Model file for the job. Use its own axes, mm. Face numbers are marked on the shaded views. A direction names the side the tool comes from. Give positions to 0.01 mm unless a question says otherwise; leave off trailing zeros. Loops run counter-clockwise (first coordinate to the right, second up) from the corner with the lowest first, then second, coordinate; pieces in that order, holes last. Notation, with made-up numbers: M 16.25,74.5 L 46.25,74.5 A7 cw 46.25,86.5 Z; hole C 50.25,36.5 d5. An arc over 180 degrees is marked long. Use CSV: the item, a comma, the result in double quotes. Start each with the question number.
(1) Slice it at B-B on z = 46. List the corners of the cut face in (x, y), and give its area (3 significant figures).
(2) Slice it at D-D on y = -16.25. State how many separate pieces and enclosed holes the cut face has, and give its area (3 significant figures).
(3) Tool access for the marked faces 1, 2 and 3: list every direction of +Z, -Z, +X, -X, +Y, -Y with a clear straight run to the whole face (end or side of a thin tool).
(4) Slice it at C-C on z = 30. List the corners of the cut face in (x, y).
(5) Flat gauge pins, fed straight in: P1, Ø1, axis at y = -7, z = 56.5, coming from the -X side; P2, Ø13.5, axis at x = 0, y = 0, coming from the +Z side; P3, Ø5.5, axis at x = 21, y = -1, coming from the -Z side; P4, Ø12, axis at y = -25, z = 60.5, coming from the -X side. Where does each tip first touch, or does it go through?
(6) Wall check: line 1 along Y through (x, z) = (0, 64.3); line 2 along Y through (x, z) = (0, 2); line 3 along Y through (x, z) = (0, 39). Give the ranges that are in metal, low to high. Write a range as from..to.
(7) Slice it at A-A on y = -32.5. List the corners of the cut face in (x, z).
```python
from build123d import *

# Parameters (mm, degrees)
SKETCH_1_R               = 25
EXTRUDE_1_DEPTH          = 4
SKETCH_2_R               = 25
SKETCH_2_R_2             = 21
EXTRUDE_2_DEPTH          = 64
EXTRUDE_START            = -6
SKETCH_3_R               = 37.5
SKETCH_3_R_2             = 21
SKETCH_3_R_3             = 2.5
EXTRUDE_3_DEPTH          = 6
FILLET_1_R               = 3
SKETCH_4_R               = 4.25
SKETCH_4_R_2             = 1.5
CUT_EXTRUDE_1_DEPTH      = 5
CUT_EXTRUDE_2_DEPTH      = 50
PATTERN_CIRCULAR_2_COUNT = 4
CUT_EXTRUDE_3_DEPTH      = 100
PATTERN_CIRCULAR_3_COUNT = 4
CUT_EXTRUDE_4_DEPTH      = 2


with BuildPart() as part:
    # 草图1 → 凸台-拉伸1 (new body)
    with BuildSketch(Plane.XY):
        Circle(SKETCH_1_R)
    extrude(amount=EXTRUDE_1_DEPTH)

    # 草图2 → 凸台-拉伸2 (add)
    with BuildSketch(Plane.XY.offset(4)):
        Circle(SKETCH_2_R)
        Circle(SKETCH_2_R_2, mode=Mode.SUBTRACT)
    extrude(amount=EXTRUDE_2_DEPTH)

    # 草图3 → 凸台-拉伸3 (add)
    with BuildSketch(Plane.XY.offset(68).offset(EXTRUDE_START)):
        Circle(SKETCH_3_R)
        Circle(SKETCH_3_R_2, mode=Mode.SUBTRACT)
        with Locations((0, 32.5)):
            Circle(SKETCH_3_R_3, mode=Mode.SUBTRACT)
        with Locations((28.145825623, 16.25)):
            Circle(SKETCH_3_R_3, mode=Mode.SUBTRACT)
        with Locations((28.145825623, -16.25)):
            Circle(SKETCH_3_R_3, mode=Mode.SUBTRACT)
        with Locations((0, -32.5)):
            Circle(SKETCH_3_R_3, mode=Mode.SUBTRACT)
        with Locations((-28.145825623, -16.25)):
            Circle(SKETCH_3_R_3, mode=Mode.SUBTRACT)
        with Locations((-28.145825623, 16.25)):
            Circle(SKETCH_3_R_3, mode=Mode.SUBTRACT)
    extrude(amount=EXTRUDE_3_DEPTH)

    # 圆角1
    fillet_1_edges = [part.edges().sort_by_distance(p)[0] for p in [
        (-25, 0, 62),
    ]]
    fillet(fillet_1_edges, radius=FILLET_1_R)

    # 草图4 → 切除-拉伸1 (cut)
    with BuildSketch(Plane(origin=(0, 0, 0), x_dir=(-1, 0, 0), z_dir=(0, 0, -1))):
        Circle(SKETCH_4_R)
        with Locations((0, 9.25)):
            Circle(SKETCH_4_R_2)
        with Locations((7.75, 0)):
            Circle(SKETCH_4_R_2)
        with Locations(Location((0, -9.25, 0), (0, 0, 180))):
            Circle(SKETCH_4_R_2)
        with Locations(Location((-7.75, 0, 0), (0, 0, 180))):
            Circle(SKETCH_4_R_2)
    extrude(amount=-CUT_EXTRUDE_1_DEPTH, mode=Mode.SUBTRACT)

    # 草图5 → 切除-拉伸2 (cut, symmetric)
    with BuildSketch(Plane(origin=(0, 0, 0), x_dir=(0, 0, -1), z_dir=(1, 0, 0))):
        Polygon((-12, 0), (-24, 6.92820323), (-24, -6.92820323), align=None)
    cut_extrude_2 = extrude(amount=CUT_EXTRUDE_2_DEPTH, both=True, mode=Mode.SUBTRACT)

    # 阵列(圆周)2: 切除-拉伸2 ×4 about axis
    pattern_circular_2_axis = Axis((0, 0, 0), (0, 0, 1))
    for i in range(1, PATTERN_CIRCULAR_2_COUNT):
        add(cut_extrude_2.rotate(pattern_circular_2_axis, i * 360 / PATTERN_CIRCULAR_2_COUNT), mode=Mode.SUBTRACT)

    # 草图7 → 切除-拉伸3 (cut)
    with BuildSketch(Plane(origin=(17.67766953, 17.67766953, 0), x_dir=(0.7071067811865487, -0.7071067811865465, 0), z_dir=(0.7071067811865465, 0.7071067811865487, 0))):
        Polygon((0, -37), (-6.92820323, -49), (6.92820323, -49), align=None)
    cut_extrude_3 = extrude(amount=-CUT_EXTRUDE_3_DEPTH, mode=Mode.SUBTRACT)

    # 阵列(圆周)3: 切除-拉伸3 ×4 about axis
    pattern_circular_3_axis = Axis((0, 0, 0), (0, 0, 1))
    for i in range(1, PATTERN_CIRCULAR_3_COUNT):
        add(cut_extrude_3.rotate(pattern_circular_3_axis, i * 360 / PATTERN_CIRCULAR_3_COUNT), mode=Mode.SUBTRACT)

    # 草图8 → 切除-拉伸4 (cut)
    with BuildSketch(Plane(origin=(0, 0, 0), x_dir=(-1, 0, 0), z_dir=(0, 0, -1))):
        with BuildLine():
            ThreePointArc((-12.374368671, -12.374368671), (-17.5, 0), (-12.374368671, 12.374368671))
            Line((-12.374368671, 12.374368671), (-14.849242405, 14.849242405))
            ThreePointArc((-14.849242405, 14.849242405), (-21, 0), (-14.849242405, -14.849242405))
            Line((-14.849242405, -14.849242405), (-12.374368671, -12.374368671))
        make_face()
        with BuildLine():
            Line((14.849242405, 14.849242405), (12.374368671, 12.374368671))
            ThreePointArc((12.374368671, 12.374368671), (16.167891819, 6.696960066), (17.5, 0))
            ThreePointArc((17.5, 0), (16.167891819, -6.696960066), (12.374368671, -12.374368671))
            Line((12.374368671, -12.374368671), (14.849242405, -14.849242405))
            ThreePointArc((14.849242405, -14.849242405), (19.401470183, -8.03635208), (21, 0))
            ThreePointArc((21, 0), (19.401470183, 8.03635208), (14.849242405, 14.849242405))
        make_face()
    extrude(amount=-CUT_EXTRUDE_4_DEPTH, mode=Mode.SUBTRACT)


solid = part.part
```
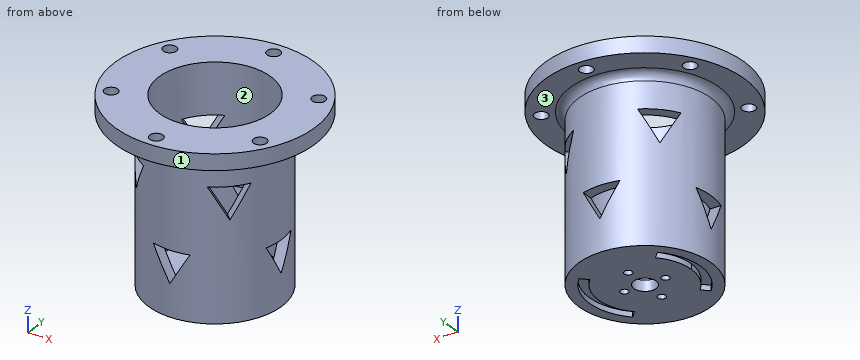
Reply:
1,outline,"M -20.97,-13.62 L -18.06,-10.71 A21 cw -18.06,10.71 L -20.97,13.62 A25 ccw Z; M -13.62,-20.97 A25 ccw 13.62,-20.97 L 10.71,-18.06 A21 cw -10.71,-18.06 Z; M -13.62,20.97 L -10.71,18.06 A21 cw 10.71,18.06 L 13.62,20.97 A25 ccw Z; M 18.06,-10.71 L 20.97,-13.62 A25 ccw 20.97,13.62 L 18.06,10.71 A21 cw Z"
1,area,"410 mm^2"
2,separate pieces,"5"
2,enclosed holes,"0"
2,area,"887 mm^2"
3,face 1,"+Z, -Z"
3,face 2,"+Z"
3,face 3,"-Z"
4,outline,"C 0,0 d50; hole C 0,0 d42"
5,P1,"stops at x = -24.14"
5,P2,"stops at z = 4"
5,P3,"stops at z = 0"
5,P4,"stops at x = -32.22"
6,line 1,"y = -37.5..-35, -30..-21, 21..30, 35..37.5"
6,line 2,"y = -25..-10.75, -7.75..-4.25, 4.25..7.75, 10.75..25"
6,line 3,"y = -25..-21, 21..25"
7,outline,"M -18.71,62 L -2.5,62 L -2.5,68 L -18.71,68 Z; M 2.5,62 L 18.71,62 L 18.71,68 L 2.5,68 Z"
